Here's how the part is built. I have some questions about the finished solid (model axes, mm). A direction names the side the tool comes from. Round coordinates to 2 decimals unless told otherwise and drop trailing zeros. Loops run counter-clockwise (first coordinate to the right, second up) from the corner with the lowest first, then second, coordinate; pieces in that order, holes last. Notation, with made-up numbers: M -22,-17 L 18,-17 A33 cw 18,16 Z; hole C -27,-22.75 d9. An arc over 180 degrees is marked long. Use a Markdown table: item, result.
from build123d import *

# Parameters (mm, degrees)
F0_W     = 300
F0_H     = 300
F1_DEPTH = 10
F2_W     = 10
F2_H     = 10
F2_W_2   = 19.925
F2_H_2   = 9.925
F2_H_3   = 19.925
F3_DEPTH = 10.001


with BuildPart() as f1:
    # F0 (on Top) → F1 (new body)
    with BuildSketch(Plane.XY):
        with Locations((150, 150)):
            Rectangle(F0_W, F0_H)
    extrude(amount=F1_DEPTH)

    # F2 (on face) → F3 (cut, through all)
    with BuildSketch(Plane.XY):
        with Locations((295, 295)):
            Rectangle(F2_W, F2_H)
        with Locations((259.9625, 295)):
            Rectangle(F2_W_2, F2_H)
        with Locations((219.9625, 295)):
            Rectangle(F2_W_2, F2_H)
        with Locations((179.9625, 295)):
            Rectangle(F2_W_2, F2_H)
        with Locations((139.9625, 295)):
            Rectangle(F2_W_2, F2_H)
        with Locations((99.9625, 295)):
            Rectangle(F2_W_2, F2_H)
        with Locations((59.9625, 295)):
            Rectangle(F2_W_2, F2_H)
        Polygon((29.925, 290), (29.925, 300), (-24.5567484915, 300), (-24.5567484915, 290), (0, 290), (0, 299.925), (10, 299.925), (10, 290), align=None)
        with Locations((5, 285)):
            Rectangle(F2_W, F2_H)
        with Locations((5, 294.9625)):
            Rectangle(F2_W, F2_H_2)
        with Locations((295, 5)):
            Rectangle(F2_W, F2_H)
        with Locations((259.9625, 5)):
            Rectangle(F2_W_2, F2_H)
        with Locations((219.9625, 5)):
            Rectangle(F2_W_2, F2_H)
        with Locations((179.9625, 5)):
            Rectangle(F2_W_2, F2_H)
        with Locations((139.9625, 5)):
            Rectangle(F2_W_2, F2_H)
        with Locations((99.9625, 5)):
            Rectangle(F2_W_2, F2_H)
        with Locations((59.9625, 5)):
            Rectangle(F2_W_2, F2_H)
        with Locations((19.9625, 5)):
            Rectangle(F2_W_2, F2_H)
        Polygon((0, 0), (10, 0), (10, 10), (10, 19.925), (0, 19.925), align=None)
        with Locations((5, 49.9625)):
            Rectangle(F2_W, F2_H_3)
        with Locations((5, 89.9625)):
            Rectangle(F2_W, F2_H_3)
        with Locations((5, 129.9625)):
            Rectangle(F2_W, F2_H_3)
        with Locations((5, 169.9625)):
            Rectangle(F2_W, F2_H_3)
        with Locations((5, 209.9625)):
            Rectangle(F2_W, F2_H_3)
        with Locations((5, 249.9625)):
            Rectangle(F2_W, F2_H_3)
    extrude(amount=F3_DEPTH, mode=Mode.SUBTRACT)


solid = f1.part
1. For pin 1 Ø3 at (y, z) = (297, 6.5) entering from -X (3 decimals); pin 2 Ø5 at (y, z) = (14, 6.5) entering from -X; pin 3 Ø2 at (x, y) = (54.5, 30.5) entering from -Z; pin 4 Ø3 at (x, z) = (2.5, 2.5) entering from +Y, each with a flat end and sliding along its axis, tell me the tip position at first contact or that it passes through.
Answer sheet:
| item | result |
|---|---|
| pin 1 | x = 29.925 |
| pin 2 | x = 10 |
| pin 3 | z = 0 |
| pin 4 | y = 280 |
2. Imagine slicing it at B-B, the plane x = 264. Write out the boundary of the cut face in (y, z), then the cut area to 3 significant figures.
Answer sheet:
| item | result |
|---|---|
| outline | M 10,0 L 290,0 L 290,10 L 10,10 Z |
| area | 2,800 mm2 |
3. Which directions (+Z, -Z, +X, -X, +Y, -Y) give clear straight access to the entire face, cutting with the end or side of a thin tool? Please do faces 5 (the face through (180, 290, 5)), 6 (the face through (290, 5, 5)), 7 (the face through (229.925, 5, 5)), 8 (the face through (10, 170, 5)).
Answer sheet:
| item | result |
|---|---|
| face 5 | +Z, -Z, +Y |
| face 6 | +Z, -Z, +X, -Y |
| face 7 | +Z, -Z, -Y |
| face 8 | +Z, -Z, -X |
4. We'd pull the mould along Y, two halves only. Please class faces 1 (the face through (140, 290, 5)), 2 (the face through (180, 10, 5)), 3 (the face through (10, 90, 5)), 4 (the face through (170, 295, 5)): +Y half, -Y half, draft (parallel to the pull), parting line (faces both ways), or undercut.
Answer sheet:
| item | result |
|---|---|
| face 1 | +Y half |
| face 2 | -Y half |
| face 3 | undercut |
| face 4 | draft |
5. Imagine slicing it at A-A, the plane y = 136.5. Write out the boundary of the cut face in (x, z), then the cut area to 3 significant figures.
Answer sheet:
| item | result |
|---|---|
| outline | M 10,0 L 300,0 L 300,10 L 10,10 Z |
| area | 2,900 mm2 |
6. I need wall thicknesses on probe 1 along Y at (x, z) = (182, 1.5); probe 2 along X at (y, z) = (42, 1). Which ranges of each line are inside material? Lowest first, please. Write a range as from..to.
Answer sheet:
| item | result |
|---|---|
| probe 1 | 10..290 |
| probe 2 | 10..300 |
